Source: CAD feature listing. Evaluate the final solid. Frame: model axes, mm. A direction names the side the tool comes from. Coordinates: 2 decimals unless noted, no trailing zeros. Loops run counter-clockwise (first coordinate to the right, second up) from the corner with the lowest first, then second, coordinate; pieces in that order, holes last.
```python
from build123d import *

# Parameters (mm, degrees)
F0_R     = 55
F0_R_2   = 51
F0_R_3   = 47
F1_DEPTH = 5
F2_DEPTH = 50
F3_DEPTH = 100
F4_R     = 10
F5_DEPTH = 25
F6_DEPTH = 25
F7_DEPTH = 25


# Not quite as in the source:
# - a fillet or chamfer that OpenCascade refuses, or shapes differently, is made with other operations: its cross-section is extruded or revolved along the edge and cut away or added


with BuildPart() as f1:
    # F0 (on Top) → F1 (new body)
    with BuildSketch(Plane.XY):
        Circle(F0_R)
        Circle(F0_R_2, mode=Mode.SUBTRACT)
        Circle(F0_R_2)
        Circle(F0_R_3, mode=Mode.SUBTRACT)
        Circle(F0_R_3)
    extrude(amount=F1_DEPTH)

    # F0 (on Top) → F2 (join)
    with BuildSketch(Plane.XY):
        Circle(F0_R_2)
        Circle(F0_R_3, mode=Mode.SUBTRACT)
    extrude(amount=F2_DEPTH)

    # F3 (add): a face of the model
    f3_faces = [f1.faces().sort_by_distance(p)[0] for p in [
        (-53.4443650814, 0, 5),
    ]]
    extrude(f3_faces, amount=F3_DEPTH)

    # F4
    f4_edges = [f1.edges().sort_by_distance(p)[0] for p in [
        (-55, 0, 0),
    ]]
    fillet(f4_edges, radius=F4_R)

    # F0 (on Top) → F5 (join)
    with BuildSketch(Plane.XY):
        Circle(F0_R)
        Circle(F0_R_2, mode=Mode.SUBTRACT)
    extrude(amount=F5_DEPTH)

    # F0 (on Top) → F6 (join)
    with BuildSketch(Plane.XY):
        Circle(F0_R)
        Circle(F0_R_2, mode=Mode.SUBTRACT)
    extrude(amount=F6_DEPTH)

    # F0 (on Top) → F7 (join)
    with BuildSketch(Plane.XY):
        Circle(F0_R)
        Circle(F0_R_2, mode=Mode.SUBTRACT)
    extrude(amount=F7_DEPTH)

    # F8: fillet of radius 7 on 1 edges, made by hand

    # F8_s1 → F8_t2 (revolve, cut)
    with BuildSketch(Plane.XZ):
        with BuildLine():
            ThreePointArc((55, 6.3245553203), (53.9160797831, 2.5828979336), (51, 0))
            Line((51, 0), (55, 0))
            Line((55, 0), (55, 6.3245553203))
        make_face()
    revolve(axis=Axis((0, 0, 0), (0, 0, 1)), mode=Mode.SUBTRACT)


solid = f1.part
```
Q1. Section query C-C on z = 18. Return the cut outline in (x, y), then the cut area to 3 significant figures.
Q2. Material intervals for line 1 along Y through (x, z) = (0, 37.5); line 2 along Y through (x, z) = (0, 1); line 3 along Z through (x, y) = (-29.5, -31.5), sorted ascending.
Q3. First-contact query: pin 1 Ø12 at (x, z) = (-35.5, 76.5) entering from -Y; pin 2 Ø1 at (x, y) = (2, 18.5) entering from +Z; pin 3 Ø4 at (x, z) = (26, 56.5) entering from -Y. Flat tips, straight axial feed; report the tip coordinate or a pass-through.
Q4. Section query A-A on y = 0. Return the cut outline in (x, z).
Q5. Draft query along X for faces 1 (the flat face through (-1, 1, 0)), 2 (the flat face through (-1, 1, 5)), 3 (the cylindrical face through (-11.923, -53.692, 54.972)). Return one class per face: released by +X, released by -X, zero draft, split by the parting line, or undercut.
Q6. Reachability of faces 4 (the flat face through (16, -49, 105)), 5 (the cylindrical face through (44.83, 14.12, 27.18)) from +Z, -Z, +X, -X, +Y, -Y: full face, straight path, thin tool, end or side. Return the list, or none.
Resolved:
1. outline: circle Ø110 at (0, 0); hole circle Ø94 at (0, 0)
1. area: 2,560 mm2
2. line 1: y = -55 to -47, 47 to 55
2. line 2: y = -52.54 to -51, -49.36 to 49.36, 51 to 52.54
2. line 3: z = 0 to 5
3. pin 1: stops at y = -46.42
3. pin 2: stops at z = 5
3. pin 3: stops at y = -49.49
4. outline: (-55, 6.32) arc R7 ccw to (-51, 0) - (-51, 2) arc R10 ccw to (-45, 0) - (45, 0) arc R10 ccw to (51, 2) - (51, 0) arc R7 ccw to (55, 6.32) - (55, 105) - (51, 105) - (51, 50) - (47, 50) - (47, 5) - (-47, 5) - (-47, 50) - (-51, 50) - (-51, 105) - (-55, 105) - close
5. face 1: zero draft
5. face 2: undercut
5. face 3: split by the parting line
6. face 4: +Z, +X, -X, +Y, -Y
6. face 5: +Z
